```python
from build123d import *

# Parameters (mm, degrees)
SKETCH1_W                                        = 3.5
SKETCH1_H                                        = 3.8
BOSS_EXTRUDE1_DEPTH                              = 1.5
CUT_EXTRUDE1_DEPTH                               = 2
F_0_9_0_9_DIAMETER_HOLE1_D                       = 0.9
F_0_9_0_9_DIAMETER_HOLE1_DEPTH                   = 3.8
CBORE_FOR_M2_HEX_HEAD_MACHINE_SCREW1_D           = 2.5
CBORE_FOR_M2_HEX_HEAD_MACHINE_SCREW1_DEPTH       = 3.8
CBORE_FOR_M2_HEX_HEAD_MACHINE_SCREW1_CBORE_D     = 4.7
CBORE_FOR_M2_HEX_HEAD_MACHINE_SCREW1_CBORE_DEPTH = 1


with BuildPart() as part:
    # Sketch1 → Revolve1 (revolve)
    with BuildSketch(Plane(origin=(0, 0, 0), x_dir=(1, 0, 0), z_dir=(0, 1, 0))):
        with Locations((1.75, -1.9)):
            Rectangle(SKETCH1_W, SKETCH1_H)
    revolve(axis=Axis((0, 0, 0), (0, 0, 1)))

    # Sketch2 → Boss-Extrude1 (add)
    with BuildSketch(Plane(origin=(0, 0, 0), x_dir=(-1, 0, 0), z_dir=(0, 0, -1))):
        with BuildLine():
            Line((-1.9, 14.1), (-2.75, 2.165063509))
            ThreePointArc((-2.75, 2.165063509), (0, 3.5), (2.75, 2.165063509))
            Line((2.75, 2.165063509), (1.9, 14.1))
            ThreePointArc((1.9, 14.1), (0, 16), (-1.9, 14.1))
        make_face()
    extrude(amount=-BOSS_EXTRUDE1_DEPTH)

    # Sketch3 → Cut-Extrude1 (cut)
    with BuildSketch(Plane.XY.offset(3.8)):
        Polygon((2.06028803, 1.324066719), (1.700436542, 1.473436651), (1.603799186, 1.850882928), (1.216441839, 1.892820449), (1.017380071, 2.227751609), (0.633898253, 2.158859191), (0.348538872, 2.424141105), (0, 2.25), (-0.348538872, 2.424141105), (-0.633898253, 2.158859191), (-1.017380071, 2.227751609), (-1.216441839, 1.892820449), (-1.603799186, 1.850882928), (-1.700436542, 1.473436651), (-2.06028803, 1.324066719), (-2.04667199, 0.934683779), (-2.34986459, 0.689982499), (-2.227098244, 0.320208386), (-2.449069097, 0), (-2.227098244, -0.320208386), (-2.34986459, -0.689982499), (-2.04667199, -0.934683779), (-2.06028803, -1.324066719), (-1.700436542, -1.473436651), (-1.603799186, -1.850882928), (-1.216441839, -1.892820449), (-1.017380071, -2.227751609), (-0.633898253, -2.158859191), (-0.348538872, -2.424141105), (0, -2.25), (0.348538872, -2.424141105), (0.633898253, -2.158859191), (1.017380071, -2.227751609), (1.216441839, -1.892820449), (1.603799186, -1.850882928), (1.700436542, -1.473436651), (2.06028803, -1.324066719), (2.04667199, -0.934683779), (2.34986459, -0.689982499), (2.227098244, -0.320208386), (2.449069097, 0), (2.227098244, 0.320208386), (2.34986459, 0.689982499), (2.04667199, 0.934683779), align=None)
    extrude(amount=-CUT_EXTRUDE1_DEPTH, mode=Mode.SUBTRACT)

    # Ø0.9 (0.9) Diameter Hole1
    with Locations(Plane(origin=(0, 0, 0), x_dir=(-1, 0, 0), z_dir=(0, 0, -1))):
        with Locations((0, 10.6), (0, 12.7), (0, 14.8), (0, 6.4), (0, 8.5), (0, 4.3)):
            Hole(F_0_9_0_9_DIAMETER_HOLE1_D / 2, depth=F_0_9_0_9_DIAMETER_HOLE1_DEPTH)

    # CBORE for M2 Hex Head Machine Screw1
    with Locations(Plane(origin=(0, 0, 0), x_dir=(-1, 0, 0), z_dir=(0, 0, -1))):
        with Locations((0, 0)):
            CounterBoreHole(CBORE_FOR_M2_HEX_HEAD_MACHINE_SCREW1_D / 2, CBORE_FOR_M2_HEX_HEAD_MACHINE_SCREW1_CBORE_D / 2, CBORE_FOR_M2_HEX_HEAD_MACHINE_SCREW1_CBORE_DEPTH, depth=CBORE_FOR_M2_HEX_HEAD_MACHINE_SCREW1_DEPTH)


solid = part.part
```
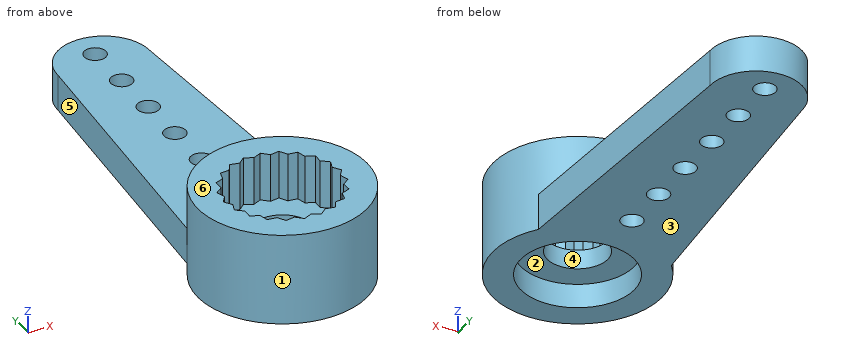
Part model, mm, in its own coordinate system. Face numbers are marked on the shaded views. A direction names the side the tool comes from. Coordinates: 2 decimals unless noted, no trailing zeros. Order: outer loops, then holes, each group sorted by start corner. A loop starts at its lowest first (then second) coordinate and runs counter-clockwise, first axis right, second up. Notation, with made-up numbers: (16, -26.75) - (67, -26.75) arc R8 ccw to (67, -21.75) - close; hole circle Ø9 at (68.5, -39). An arc over 180 degrees is marked (long way). Return JSON: item names as keys, results as strings. Group by question number.
Item 1: Which spindle directions (+Z, -Z, +X, -X, +Y, -Y) get a long thin tool onto all of the face, cutting with end or side? Do the marked faces 1, 2 and 3. Say none if no direction does.
Item 2: Pull direction X, two halves, no side cores. Call the marked faces 4, 5 and 6: pulls with the +X half, pulls with the -X half, needs draft (parallel to the pull), parting line crosses it, or undercut.
Item 3: Pin check, flat tips, straight feed: pin 1 (3 mm diameter, centred on x = 0, y = 0, fed in from -Z); pin 2 (4 mm diameter, centred on x = 0.5, y = 11.5, fed in from -Z); pin 3 (4 mm diameter, centred on x = 0, y = 0, fed in from +Z); pin 4 (2 mm diameter, centred on x = 1.5, y = 14, fed in from +Z). Stop position of each tip, or through.
Item 4: Cut at B-B (y = 14.8). List the corners of the cut face in (x, z).
Item 5: Cut at C-C (y = 8.5). List the corners of the cut face in (x, z), plus the area to 3 significant figures.
Item 6: Cut at D-D (x = 3). List the corners of the cut face in (y, z).
Item 7: Cut at A-A (z = 0.8). List the corners of the cut face in (x, y), plus the area to 3 significant figures.
Item 8: Drill centre lines: probe 1 along Z at (x, y) = (1.25, 6.5); probe 2 along Z at (x, y) = (2.25, 0); probe 3 along Y at (x, z) = (-1.5, 2.7). Where is each one in solid material? Low to high. Write a range as from..to.
Check values:
{
 "1": {"face 1": "+Z", "face 2": "-Z", "face 3": "-Z, +X, -X, +Y, -Y"},
 "2": {"face 4": "undercut", "face 5": "pulls with the -X half", "face 6": "needs draft"},
 "3": {"pin 1": "stops at z = 1", "pin 2": "stops at z = 0", "pin 3": "stops at z = 1.8", "pin 4": "stops at z = 1.5"},
 "4": {"outline": "(-1.77, 0) - (-0.45, 0) - (-0.45, 1.5) - (-1.77, 1.5) - close; (0.45, 0) - (1.77, 0) - (1.77, 1.5) - (0.45, 1.5) - close"},
 "5": {"outline": "(-2.3, 0) - (-0.45, 0) - (-0.45, 1.5) - (-2.3, 1.5) - close; (0.45, 0) - (2.3, 0) - (2.3, 1.5) - (0.45, 1.5) - close", "area": "5.55 mm2"},
 "6": {"outline": "(-1.8, 0) - (1.8, 0) - (1.8, 3.8) - (-1.8, 3.8) - close"},
 "7": {"outline": "(-2.75, 2.17) arc R3.5 ccw (long way) to (2.75, 2.17) - (1.9, 14.1) arc R1.9 ccw to (-1.9, 14.1) - close; hole circle Ø4.7 at (0, 0); hole circle Ø0.9 at (0, 4.3); hole circle Ø0.9 at (0, 6.4); hole circle Ø0.9 at (0, 8.5); hole circle Ø0.9 at (0, 10.6); hole circle Ø0.9 at (0, 12.7); hole circle Ø0.9 at (0, 14.8)", "area": "73.4 mm2"},
 "8": {"probe 1": "z = 0..1.5", "probe 2": "z = 1..1.8", "probe 3": "y = -3.16..-1.86, 1.86..3.16"}
}
